Source: CAD feature listing. Evaluate the final solid. Frame: model axes, mm. Give positions to 0.01 mm unless a question says otherwise; leave off trailing zeros. Order: outer loops, then holes, each group sorted by start corner. A loop starts at its lowest first (then second) coordinate and runs counter-clockwise, first axis right, second up. Notation, with made-up numbers: (29.25, 29.5) - (81.25, 29.5) arc R17 ccw to (81.25, 52.5) - close; hole circle Ø5 at (9.25, -34). An arc over 180 degrees is marked (long way). One line per item, written item: value. Start each with the question number.
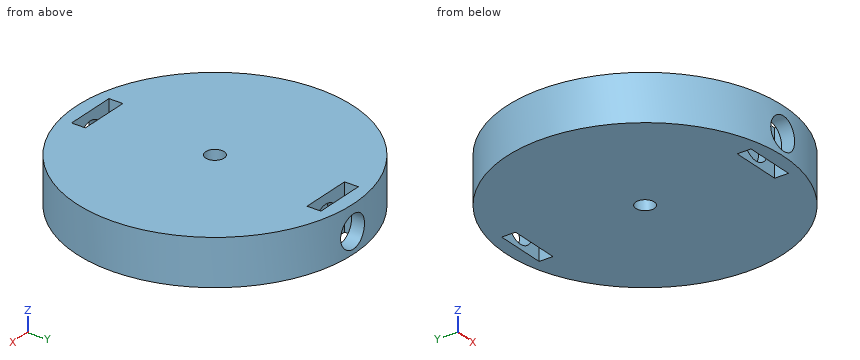
from build123d import *

# Parameters (mm, degrees)
SKETCH1_R           = 30
BOSS_EXTRUDE1_DEPTH = 10
SKETCH10_R          = 3.5
CUT_EXTRUDE6_DEPTH  = 8
SKETCH23_W          = 11
SKETCH23_H          = 3
CUT_EXTRUDE8_DEPTH  = 10
SKETCH24_R          = 2
CUT_EXTRUDE9_DEPTH  = 10


with BuildPart() as part:
    # Sketch1 → Boss-Extrude1 (new body)
    with BuildSketch(Plane.XY):
        Circle(SKETCH1_R)
    extrude(amount=BOSS_EXTRUDE1_DEPTH)

    # Sketch10 → Cut-Extrude6 (cut)
    with BuildSketch(Plane(origin=(0, -30, 0), x_dir=(-1, 0, 0), z_dir=(0, -1, 0))):
        with Locations(Location((0, -4.5, 0), (0, 0, 90))):
            Circle(SKETCH10_R)
    cut_extrude6 = extrude(amount=-CUT_EXTRUDE6_DEPTH, mode=Mode.SUBTRACT)

    # Mirror2: Cut-Extrude6 across plane
    add(cut_extrude6.mirror(Plane.ZX), mode=Mode.SUBTRACT)

    # Sketch23 → Cut-Extrude8 (cut)
    with BuildSketch(Plane(origin=(0, 0, 0), x_dir=(-1, 0, 0), z_dir=(0, 0, -1))):
        with Locations((0, 25.5)):
            Rectangle(SKETCH23_W, SKETCH23_H)
    cut_extrude8 = extrude(amount=-CUT_EXTRUDE8_DEPTH, mode=Mode.SUBTRACT)

    # Mirror3: Cut-Extrude8 across plane
    add(cut_extrude8.mirror(Plane.ZX), mode=Mode.SUBTRACT)

    # Sketch24 → Cut-Extrude9 (cut)
    with BuildSketch(Plane(origin=(0, 0, 0), x_dir=(-1, 0, 0), z_dir=(0, 0, -1))):
        Circle(SKETCH24_R)
    extrude(amount=-CUT_EXTRUDE9_DEPTH, mode=Mode.SUBTRACT)


solid = part.part
1. Ray query, L1, parallel to Y at x = 0, z = 5.75; L2, parallel to Z at x = 0, y = 27.8; L3, parallel to Y at x = -5, z = 8.5. Return the intervals inside material, ascending.
2. Section B-B on y = 0. Return the cut outline in (x, z), then the cut area to 3 significant figures.
3. Contact query for flat-ended pins moving along their axis: pin 1 Ø1.5 at (y, z) = (-15, 7.5) entering from +X; pin 2 Ø4 at (x, z) = (0, 4.5) entering from -Y; pin 3 Ø1 at (y, z) = (-23.5, 3) entering from -X. Output: stop coordinate, or through.
4. Section C-C on z = 4. Return the cut outline in (x, y), then the cut area to 3 significant figures.
5. Section D-D on y = -12.5. Return the cut outline in (x, z), then the cut area to 3 significant figures.
6. Section A-A on x = 0. Count the separate pieces of the cut face and the enclosed holes in it, then the cut area to 3 significant figures.
Data:
1. L1: y = -22 to -2, 2 to 22
1. L2: z = 0 to 1, 8 to 10
1. L3: y = -29.58 to -27, -24 to 24, 27 to 29.58
2. outline: (-30, 0) - (-2, 0) - (-2, 10) - (-30, 10) - close; (2, 0) - (30, 0) - (30, 10) - (2, 10) - close
2. area: 560 mm2
3. pin 1: stops at x = 26.4
3. pin 2: stops at y = -22
3. pin 3: stops at x = -19.26
4. outline: (-5.5, -27) - (-5.5, -24) - (-3.46, -24) - (-3.46, -22) - (3.46, -22) - (3.46, -24) - (5.5, -24) - (5.5, -27) - (3.46, -27) - (3.46, -29.8) arc R30 ccw to (3.46, 29.8) - (3.46, 27) - (5.5, 27) - (5.5, 24) - (3.46, 24) - (3.46, 22) - (-3.46, 22) - (-3.46, 24) - (-5.5, 24) - (-5.5, 27) - (-3.46, 27) - (-3.46, 29.8) arc R30 ccw to (-3.46, -29.8) - (-3.46, -27) - close; hole circle Ø4 at (0, 0)
4. area: 2,680 mm2
5. outline: (-27.27, 0) - (27.27, 0) - (27.27, 10) - (-27.27, 10) - close
5. area: 545 mm2
6. separate pieces: 6
6. enclosed holes: 0
6. area: 430 mm2
